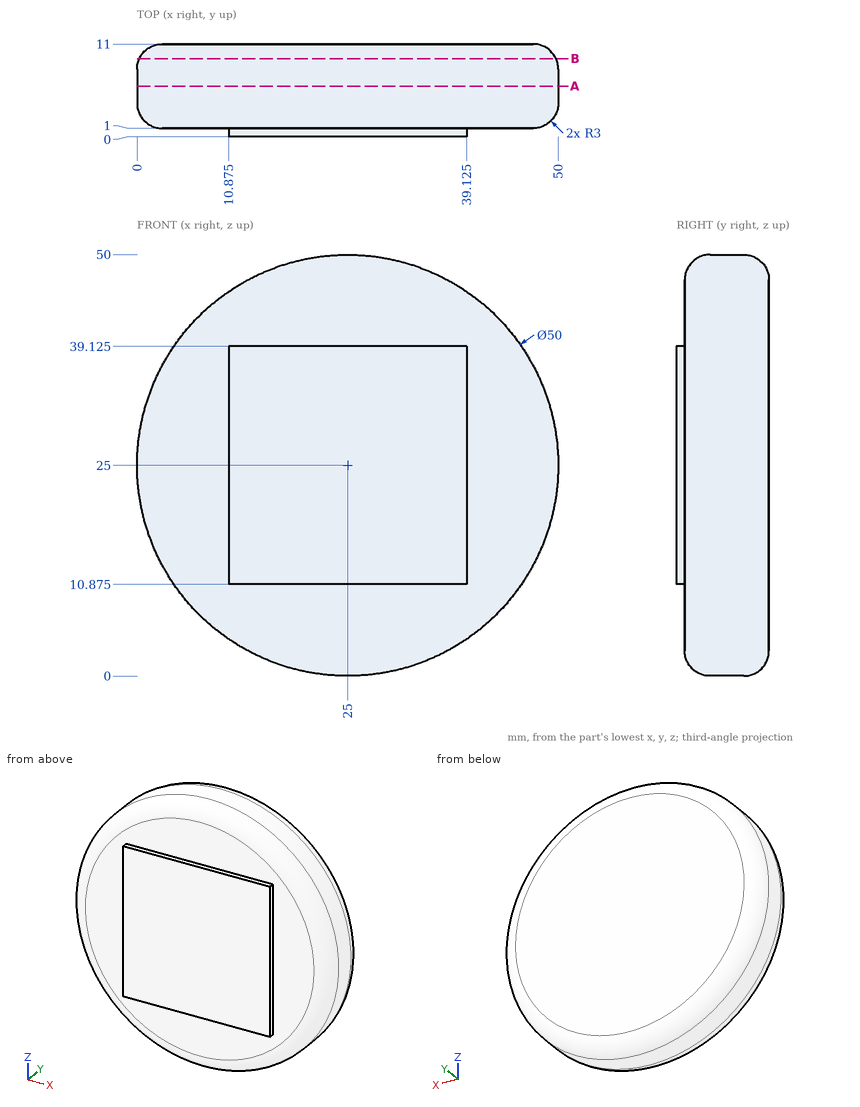
Check sheet for the drawn part. Datum: minimum x, y, z corner. Units: mm. Round coordinates to 2 decimals unless told otherwise and drop trailing zeros. Order: outer loops, then holes, each group sorted by start corner. A loop starts at its lowest first (then second) coordinate and runs counter-clockwise, first axis right, second up.
1. Section check B-B on y = 9.25. Record the cut outline in (x, z).
Final values:
outline: circle Ø49.45 at (25, 25)
2. Section check A-A on y = 6. Record the cut outline in (x, z).
Final values:
outline: circle Ø50 at (25, 25)
3. Go/stop test with flat-tipped pins: P1, Ø4, axis at x = 39.5, z = 45, coming from the -Y side; P2, Ø3, axis at y = 8.5, z = 21, coming from the +X side; P3, Ø4, axis at x = 44, y = 8, coming from the -Z side. Record where each tip stops, or that it passes through.
Final values:
P1: stops at y = 1.08
P2: stops at x = 49.87
P3: stops at z = 6.67
4. Thickness scan on L1, parallel to Y at x = 29, z = 6; L2, parallel to Z at x = 33.5, y = 9.5; L3, parallel to Y at x = 48.5, z = 21. Record the ranges inside material, lowest first.
Final values:
L1: y = 1 to 11
L2: z = 1.92 to 48.08
L3: y = 1.63 to 10.37
